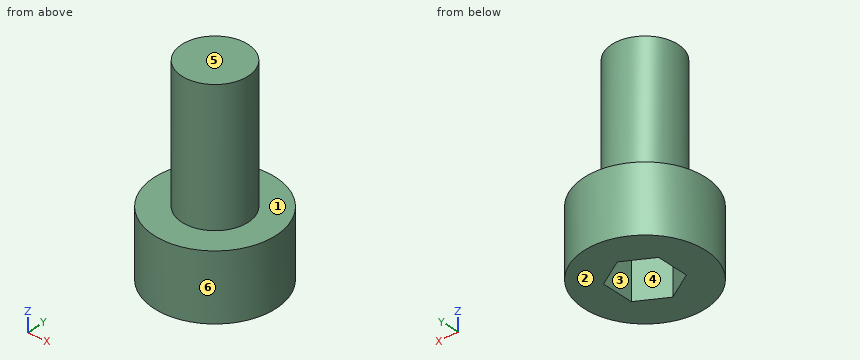
from build123d import *

# Parameters (mm, degrees)
SKETCH1_R          = 1.5
EXTRUDE1_DEPTH     = 6
SKETCH6_R          = 2.75
EXTRUDE2_DEPTH     = 3
CUT_EXTRUDE1_DEPTH = 1.875


with BuildPart() as part:
    # Sketch1 → Extrude1 (new body)
    with BuildSketch(Plane.XY):
        Circle(SKETCH1_R)
    extrude(amount=-EXTRUDE1_DEPTH)

    # Sketch6 → Extrude2 (add)
    with BuildSketch(Plane(origin=(0, 0, -6), x_dir=(-1, 0, 0), z_dir=(0, 0, -1))):
        Circle(SKETCH6_R)
    extrude(amount=EXTRUDE2_DEPTH)

    # Sketch7 → Cut-Extrude1 (cut)
    with BuildSketch(Plane(origin=(0, 0, -9), x_dir=(-1, 0, 0), z_dir=(0, 0, -1))):
        Polygon((0, 1.443375673), (-1.25, 0.721687836), (-1.25, -0.721687836), (0, -1.443375673), (1.25, -0.721687836), (1.25, 0.721687836), align=None)
    extrude(amount=-CUT_EXTRUDE1_DEPTH, mode=Mode.SUBTRACT)


solid = part.part
Read the model definition and answer for the solid it produces. Units are mm, in the model's axes. Face numbers are marked on the shaded views. A direction names the side the tool comes from. Round coordinates to 2 decimals unless told otherwise and drop trailing zeros. Order: outer loops, then holes, each group sorted by start corner. A loop starts at its lowest first (then second) coordinate and runs counter-clockwise, first axis right, second up. Notation, with made-up numbers: (69.5, 79.5) - (85.5, 79.5) arc R12 ccw to (85.5, 95.5) - close; hole circle Ø1 at (-24.75, 43.25). An arc over 180 degrees is marked (long way). Use one line per item in the form item = value. Start each with the question number.
(1) The part is cut by section A-A (y = 0). Give the vertices of the cut face in (x, z) (3 decimals), then the cut area to 3 significant figures.
(2) Find the intervals of material crossed by line 1 along X through (y, z) = (0.1, -7.25); line 2 along X through (y, z) = (0.05, -5.5); line 3 along Z through (x, y) = (0.35, 2.1), in increasing order. Write a range as from..to.
(3) For the marked faces 1 and 2, determine the directions among +Z, -Z, +X, -X, +Y, -Y from which every point of the face is accessible in a straight line to the end or side of a thin tool.
(4) Determine the mould class of the marked faces 3, 4, 5 and 6 for opening direction X: +X half, -X half, draft (parallel to the pull), parting line (faces both ways), or undercut.
(5) The part is cut by section D-D (x = -2.35). Give the vertices of the cut face in (y, z).
(6) The part is cut by section C-C (z = -5.25). Give the vertices of the cut face in (x, y).
(7) The part is cut by section B-B (x = -1.15). Give the vertices of the cut face in (y, z) (3 decimals), then the cut area to 3 significant figures.
(8) Flat-ended cylindrical pins translate along their axes: pin 1 Ø1 at (y, z) = (1.5, -1.5) entering from -X; pin 2 Ø1.2 at (x, y) = (0, 0) entering from -Z (3 decimals); pin 3 Ø1 at (x, z) = (-1.5, -3.5) entering from +Y. Find the tip coordinate at first contact, or state that the pin passes through.
Checked values:
q1.outline = (-2.75, -9) - (-1.25, -9) - (-1.25, -7.125) - (1.25, -7.125) - (1.25, -9) - (2.75, -9) - (2.75, -6) - (1.5, -6) - (1.5, 0) - (-1.5, 0) - (-1.5, -6) - (-2.75, -6) - close
q1.area = 29.8 mm^2
q2.line_1 = -2.75..-1.25, 1.25..2.75
q2.line_2 = -1.5..1.5
q2.line_3 = -9..-6
q3.face_1 = +Z
q3.face_2 = -Z, +X, -X, +Y, -Y
q4.face_3 = undercut
q4.face_4 = undercut
q4.face_5 = draft
q4.face_6 = parting line
q5.outline = (-1.43, -9) - (1.43, -9) - (1.43, -6) - (-1.43, -6) - close
q6.outline = circle Ø3 at (0, 0)
q7.outline = (-2.498, -9) - (-0.779, -9) - (-0.779, -7.125) - (0.779, -7.125) - (0.779, -9) - (2.498, -9) - (2.498, -6) - (0.963, -6) - (0.963, 0) - (-0.963, 0) - (-0.963, -6) - (-2.498, -6) - close
q7.area = 23.6 mm^2
q8.pin_1 = -1.12
q8.pin_2 = -7.125
q8.pin_3 = 1.12
